Could you check a few things on this model? Use its own coordinates, in mm. Round coordinates to 2 decimals unless told otherwise and drop trailing zeros. Loops run counter-clockwise (first coordinate to the right, second up) from the corner with the lowest first, then second, coordinate; pieces in that order, holes last. Notation, with made-up numbers: M 17.25,36.25 L 53.25,36.25 A15 cw 53.25,44.25 Z; hole C 37,-4 d5. An arc over 180 degrees is marked long. One line per item, written item: value. Start each with the question number.
Q1. Imagine slicing it at A-A (y = 17). Give the number of separate pieces and of enclosed holes in the cut face, then the cut area to 3 significant figures.
Q2. Thinking about a two-plate mould opening in X: for faces 1 (the face through (-43.66, 12, 1)), 2 (the face through (-12.26, 12.42, 27.99)), 3 (the face through (43.66, 12, 1)), which applies, released by +X, released by -X, zero draft, split by the parting line, or undercut?
Q3. Imagine slicing it at D-D (x = -26.5). Please give me the cut outline in (y, z), then the cut area to 3 significant figures.
Q4. Imagine slicing it at C-C (z = 1). Please give me the cut outline in (x, y), then the cut area to 3 significant figures.
Q5. Imagine slicing it at B-B (x = -12). Please give me the cut outline in (y, z), then the cut area to 3 significant figures.
Q6. I'm going to push a flat-ended pin straight in: pin 1 Ø20 at (x, z) = (-30.66, 52.25) entering from -Y. Where does the tip first touch, or does it pass through?
Q7. Please list where these lines run through material, in increasing order: line 1 along Z through (x, y) = (-9.5, 5); line 2 along Z through (x, y) = (-27.5, 4); line 3 along X through (y, z) = (10, 52.25).
from build123d import *

# Parameters (mm, degrees)
SKETCH2_W           = 87.32
SKETCH2_H           = 129.5
BOSS_EXTRUDE1_DEPTH = 24.5
SKETCH3_R           = 11
CUT_EXTRUDE1_DEPTH  = 25.5
LPATTERN1_COUNT     = 5
LPATTERN1_PITCH     = 23


with BuildPart() as part:
    # Sketch2 → Boss-Extrude1 (new body)
    with BuildSketch(Plane(origin=(0, 0, 0), x_dir=(1, 0, 0), z_dir=(0, 1, 0))):
        Rectangle(SKETCH2_W, SKETCH2_H)
    extrude(amount=BOSS_EXTRUDE1_DEPTH)

    # Sketch3 → Cut-Extrude1 (cut, through all)
    with BuildSketch(Plane(origin=(0, 24.5, 0), x_dir=(1, 0, 0), z_dir=(0, 1, 0))):
        with Locations((-30.66, 39.75)):
            Circle(SKETCH3_R)
        with Locations((-9.875390309, 51.75)):
            Circle(SKETCH3_R)
    cut_extrude1 = extrude(amount=-CUT_EXTRUDE1_DEPTH, mode=Mode.SUBTRACT)

    # LPattern1: Cut-Extrude1 ×5
    with Locations(*[(0, 0, i * LPATTERN1_PITCH) for i in range(1, LPATTERN1_COUNT)]):
        add(cut_extrude1, mode=Mode.SUBTRACT)


solid = part.part
Report:
1. separate pieces: 1
1. enclosed holes: 10
1. area: 7,510 mm²
2. face 1: released by -X
2. face 2: undercut
2. face 3: released by +X
3. outline: M 0,-64.75 L 24.5,-64.75 L 24.5,-49.93 L 0,-49.93 Z; M 0,-29.57 L 24.5,-29.57 L 24.5,-26.93 L 0,-26.93 Z; M 0,-6.57 L 24.5,-6.57 L 24.5,-3.93 L 0,-3.93 Z; M 0,16.43 L 24.5,16.43 L 24.5,19.07 L 0,19.07 Z; M 0,39.43 L 24.5,39.43 L 24.5,42.07 L 0,42.07 Z; M 0,62.43 L 24.5,62.43 L 24.5,64.75 L 0,64.75 Z
3. area: 678 mm²
4. outline: M -43.66,0 L -40.33,0 L -40.33,24.5 L -43.66,24.5 Z; M -20.99,0 L -18.56,0 L -18.56,24.5 L -20.99,24.5 Z; M -1.19,0 L 43.66,0 L 43.66,24.5 L -1.19,24.5 Z
4. area: 1,240 mm²
5. outline: M 0,-64.75 L 24.5,-64.75 L 24.5,-62.54 L 0,-62.54 Z; M 0,-40.96 L 24.5,-40.96 L 24.5,-39.54 L 0,-39.54 Z; M 0,-17.96 L 24.5,-17.96 L 24.5,-16.54 L 0,-16.54 Z; M 0,5.04 L 24.5,5.04 L 24.5,6.46 L 0,6.46 Z; M 0,28.04 L 24.5,28.04 L 24.5,29.46 L 0,29.46 Z; M 0,51.04 L 24.5,51.04 L 24.5,64.75 L 0,64.75 Z
5. area: 528 mm²
6. pin 1: passes through
7. line 1: z = -64.75 to -62.74, -40.76 to -39.74, -17.76 to -16.74, 5.24 to 6.26, 28.24 to 29.26, 51.24 to 64.75
7. line 2: z = -64.75 to -50.29, -29.21 to -27.29, -6.21 to -4.29, 16.79 to 18.71, 39.79 to 41.71, 62.79 to 64.75
7. line 3: x = -43.66 to -41.66, -19.66 to 43.66
